```python
from build123d import *

# Parameters (mm, degrees)
F0_R     = 25
F0_R_2   = 3
F1_DEPTH = 7
F2_R     = 12
F3_DEPTH = 15
F4_SIZE  = 1


# Not quite as in the source:
# - a fillet or chamfer that OpenCascade refuses, or shapes differently, is made with other operations: its cross-section is extruded or revolved along the edge and cut away or added


with BuildPart() as f1:
    # F0 (on Top) → F1 (new body)
    with BuildSketch(Plane.XY):
        Circle(F0_R)
        with Locations((-13, -13)):
            Circle(F0_R_2, mode=Mode.SUBTRACT)
        with Locations((13, -13)):
            Circle(F0_R_2, mode=Mode.SUBTRACT)
        with Locations((-13, 13)):
            Circle(F0_R_2, mode=Mode.SUBTRACT)
        with Locations((13, 13)):
            Circle(F0_R_2, mode=Mode.SUBTRACT)
    extrude(amount=F1_DEPTH)

    # F2 (on face) → F3 (join)
    with BuildSketch(Plane.XY.offset(7)):
        Circle(F2_R)
    extrude(amount=F3_DEPTH)

    # F4
    f4_edges = [f1.edges().sort_by_distance(p)[0] for p in [
        (-12, 0, 22),
        (-25, 0, 7),
        (-25, 0, 0),
    ]]
    chamfer(f4_edges, length=F4_SIZE)

    # F5: chamfer of 3 on 4 edges, made by hand

    # F5_s1 → F5_t2 (revolve, cut)
    with BuildSketch(Plane.XZ.offset(13)):
        Polygon((-7, 7), (-10, 4), (-10, 7), align=None)
    revolve(axis=Axis((-13, -13, 7), (0, 0, 1)), mode=Mode.SUBTRACT)

    # F5_s3 → F5_t4 (revolve, cut)
    with BuildSketch(Plane.XZ.offset(13)):
        Polygon((19, 7), (16, 4), (16, 7), align=None)
    revolve(axis=Axis((13, -13, 7), (0, 0, 1)), mode=Mode.SUBTRACT)

    # F5_s5 → F5_t6 (revolve, cut)
    with BuildSketch(Plane.XZ.offset(-13)):
        Polygon((19, 7), (16, 4), (16, 7), align=None)
    revolve(axis=Axis((13, 13, 7), (0, 0, 1)), mode=Mode.SUBTRACT)

    # F5_s7 → F5_t8 (revolve, cut)
    with BuildSketch(Plane.XZ.offset(-13)):
        Polygon((-7, 7), (-10, 4), (-10, 7), align=None)
    revolve(axis=Axis((-13, 13, 7), (0, 0, 1)), mode=Mode.SUBTRACT)


solid = f1.part
```
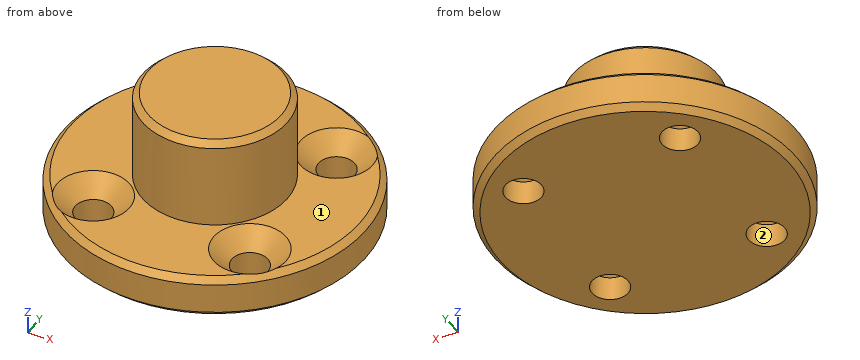
Geometry: final body of the model. Coordinates: model frame, mm. Face numbers are marked on the shaded views. A direction names the side the tool comes from. Coordinates: 2 decimals unless noted, no trailing zeros. Write each loop counter-clockwise with the first axis right and the second up, starting at its lowest first coordinate (ties: lowest second). Pieces come first, ordered by that corner, then holes. Notation, with made-up numbers: M 6.5,55 L 62.5,55 A25 ccw 62.5,79 Z; hole C 2.25,49 d1. An arc over 180 degrees is marked long. Use CSV: the item, a comma, the result in double quotes. Start each with the question number.
1. Cut plane D-D on x = 13. Count the separate pieces of the cut face and the enclosed holes in it, plus the area to 3 significant figures.
2. Ray query, probe 1 along Y at (x, z) = (-13, 1); probe 2 along Z at (x, y) = (8, 9.5); probe 3 along Y at (x, z) = (-13.5, 3.25). Return the intervals inside material, ascending.
3. Reachability of the marked faces 1 and 2 from +Z, -Z, +X, -X, +Y, -Y: full face, straight path, thin tool, end or side. Return the list, or none.
4. First-contact query: P1, Ø9.5, axis at x = 13, y = -13, coming from the +Z side; P2, Ø10, axis at x = -2, z = 15.5, coming from the +Y side; P3, Ø10, axis at y = -7.5, z = 12.5, coming from the +X side. Flat tips, straight axial feed; report the tip coordinate or a pass-through.
5. Cut plane A-A on z = 2.5. Return the cut outline in (x, y), plus the area to 3 significant figures.
6. Cut plane B-B on y = 0. Return the cut outline in (x, z).
Entries:
1,separate pieces,"3"
1,enclosed holes,"0"
1,area,"195 mm²"
2,probe 1,"-21.35 to -16, -10 to 10, 16 to 21.35"
2,probe 2,"0 to 7"
2,probe 3,"-21.04 to -15.96, -10.04 to 10.04, 15.96 to 21.04"
3,face 1,"+Z"
3,face 2,"+Z, -Z"
4,P1,"z = 5.75"
4,P2,"y = 12"
4,P3,"x = 11.74"
5,outline,"C 0,0 d50; hole C -13,-13 d6; hole C -13,13 d6; hole C 13,-13 d6; hole C 13,13 d6"
5,area,"1,850 mm²"
6,outline,"M -25,1 L -24,0 L 24,0 L 25,1 L 25,6 L 24,7 L 12,7 L 12,21 L 11,22 L -11,22 L -12,21 L -12,7 L -24,7 L -25,6 Z"
